from build123d import *

# Parameters (mm, degrees)
SKETCH1_W           = 22.5
SKETCH1_H           = 37.5
SKETCH1_W_2         = 7.5
SKETCH1_H_2         = 7.5
BOSS_EXTRUDE1_DEPTH = 5
CUT_EXTRUDE1_DEPTH  = 54.531532763


with BuildPart() as part:
    # Sketch1 → Boss-Extrude1 (new body)
    with BuildSketch(Plane(origin=(0, 0, 0), x_dir=(1, 0, 0), z_dir=(0, 1, 0))):
        Polygon((-11.25, 3.75), (-11.25, 11.25), (-18.75, 11.25), (-18.75, 26.25), (-26.25, 26.25), (-26.25, 3.75), align=None)
        Rectangle(SKETCH1_W, SKETCH1_H)
        with Locations((0, 22.5)):
            Rectangle(SKETCH1_W_2, SKETCH1_H_2)
        Polygon((26.25, 11.25), (11.25, 11.25), (11.25, 3.75), (18.75, 3.75), (18.75, -11.25), (33.75, -11.25), (33.75, -3.75), (26.25, -3.75), align=None)
        Polygon((11.25, -18.75), (3.75, -18.75), (3.75, -41.25), (18.75, -41.25), (18.75, -33.75), (11.25, -33.75), align=None)
        Polygon((-11.25, -18.75), (-11.25, -11.25), (-18.75, -11.25), (-18.75, -26.25), (-26.25, -26.25), (-26.25, -33.75), (-11.25, -33.75), align=None)
    extrude(amount=BOSS_EXTRUDE1_DEPTH)

    # Sketch2 → Cut-Extrude1 (cut, through all)
    with BuildSketch(Plane(origin=(0, 5, 0), x_dir=(1, 0, 0), z_dir=(0, 1, 0))):
        Polygon((0, 5.75), (-3.625, 9.375), (-5.625, 7.375), (-2, 3.75), (-5.625, 0.125), (-3.625, -1.875), (0, 1.75), (3.625, -1.875), (5.625, 0.125), (2, 3.75), (5.625, 7.375), (3.625, 9.375), align=None)
    extrude(amount=-CUT_EXTRUDE1_DEPTH, mode=Mode.SUBTRACT)


solid = part.part
CAD build for the part. Positions are in the model's coordinates, mm. A direction names the side the tool comes from. Coordinates: 2 decimals unless noted, no trailing zeros. Loops run counter-clockwise (first coordinate to the right, second up) from the corner with the lowest first, then second, coordinate; pieces in that order, holes last. Notation, with made-up numbers: (49.25, -2.75) - (80.25, -2.75) arc R19 ccw to (80.25, 17.25) - close; hole circle Ø10 at (45.5, 58.5). An arc over 180 degrees is marked (long way). Use one line per item in the form item = value. Start each with the question number.
1) Flat gauge pins, fed straight in: pin 1 (3 mm diameter, centred on x = -1, y = 3, fed in from +Z); pin 2 (2.5 mm diameter, centred on y = 2, z = -19, fed in from +X); pin 3 (1.5 mm diameter, centred on y = 1.5, z = -1.5, fed in from +X). Where does each tip first touch, or does it go through?
2) Band-saw the part on C-C (x = -7). Give the cut face in (y, z).
3) Band-saw the part on D-D (z = 37). Give the cut face in (x, y), and give its area (3 significant figures).
4) Tool access for faces 5 (the face through (11.25, 2, -15)), 6 (the face through (3.79, 2.54, -5.54)), 7 (the face through (-15, 2, 11.25)), 8 (the face through (15, 2, 33.75)), 9 (the face through (-26.25, 2, 30)): list every direction of +Z, -Z, +X, -X, +Y, -Y with a clear straight run to the whole face (end or side of a thin tool).
5) Band-saw the part on B-B (x = -17.5). Give the cut face in (y, z).
6) Two-plate mould, pull along X, no slides. Class faces 1 (the face through (18.75, 2, 38)), 2 (the face through (-11.25, 2, -15)), 3 (the face through (-15, 2, -11.25)), 4 (the face through (11, 2, 41.25)): +X half, -X half, draft (parallel to the pull), parting line (faces both ways), or undercut.
7) Band-saw the part on A-A (z = 6). Give the cut face in (x, y).
8) Drill centre lines: L1, parallel to Z at x = -23, y = 0.7; L2, parallel to X at y = 2.1, z = 7; L3, parallel to X at y = 2.05, z = -21. Where is each one in solid material? Low to high. Write a range as from..to.
Check values:
q1.pin_1 = 18.75
q1.pin_2 = 11.25
q1.pin_3 = 26.25
q2.outline = (0, -18.75) - (5, -18.75) - (5, 18.75) - (0, 18.75) - close
q3.outline = (3.75, 0) - (18.75, 0) - (18.75, 5) - (3.75, 5) - close
q3.area = 75.0 mm2
q4.face_5 = -Z, +X, +Y, -Y
q4.face_6 = +Y, -Y
q4.face_7 = -X, +Y, -Y
q4.face_8 = +X, +Y, -Y
q4.face_9 = +Z, -Z, -X, +Y, -Y
q5.outline = (0, -11.25) - (5, -11.25) - (5, -3.75) - (0, -3.75) - close; (0, 11.25) - (5, 11.25) - (5, 33.75) - (0, 33.75) - close
q6.face_1 = +X half
q6.face_2 = undercut
q6.face_3 = undercut
q6.face_4 = draft
q7.outline = (-11.25, 0) - (11.25, 0) - (11.25, 5) - (-11.25, 5) - close; (18.75, 0) - (33.75, 0) - (33.75, 5) - (18.75, 5) - close
q8.L1 = -26.25..-3.75, 26.25..33.75
q8.L2 = -11.25..11.25, 18.75..33.75
q8.L3 = -26.25..-18.75, -3.75..3.75
